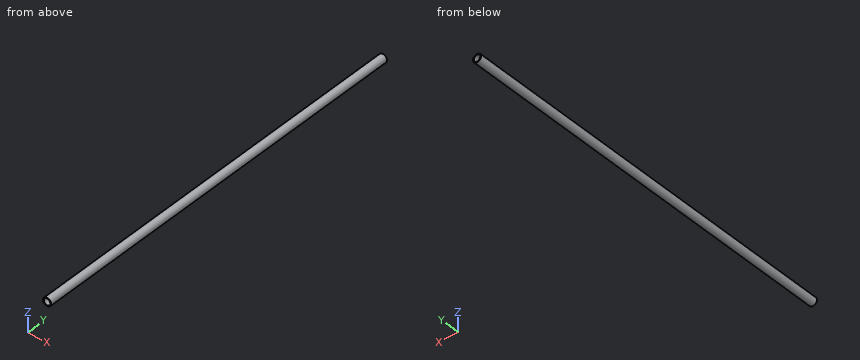
from build123d import *

# Parameters (mm, degrees)
CYLINDER_R          = 16.7005
CYLINDER_DEPTH      = 1609.72
CYLINDER_ROLL_ANGLE = 90
THICKNESS001_T      = -3.3782


with BuildPart() as part:
    # Cylinder → Cylinder (new body)
    with BuildSketch(Plane.XY):
        Circle(CYLINDER_R)
    extrude(amount=CYLINDER_DEPTH)


with BuildPart() as part_1:
    # Cylinder roll: moved
    add(part.part.rotate(Axis((0, 0, 0), (1, 0, 0)), CYLINDER_ROLL_ANGLE))


with BuildPart() as part_2:
    # Cylinder placement: moved
    add(part_1.part)

    # Thickness001
    thickness001_openings = [part_2.faces().sort_by_distance(p)[0] for p in [
        (0, 0, 0),
        (0, -1609.72, 0),
    ]]
    offset(amount=THICKNESS001_T, openings=thickness001_openings)


solid = part_2.part
Work out the finished part from the listing and answer in its coordinate system (mm). Round coordinates to 2 decimals unless told otherwise and drop trailing zeros. Order: outer loops, then holes, each group sorted by start corner. A loop starts at its lowest first (then second) coordinate and runs counter-clockwise, first axis right, second up. Notation, with made-up numbers: M -20.75,87.25 L 38.25,87.25 A14 ccw 38.25,92.25 Z; hole C -35,7.5 d2. An arc over 180 degrees is marked long. Put each result on its own line as item: value. Start each with the question number.
Q1. Straight lines are drawn through the part: L1, parallel to Z at x = 0, y = -679; L2, parallel to Z at x = -2.5, y = -1477; L3, parallel to X at y = -1381, z = 7. For each, find the intervals that lie inside material, in ascending order. Write a range as [from, to].
Q2. Flat-ended cylindrical pins translate along their axes: pin 1 (10 mm diameter, centred on x = 4, z = 2.5, fed in from +Y); pin 2 (12 mm diameter, centred on y = -988.5, z = -6.5, fed in from +X); pin 3 (2 mm diameter, centred on y = -500.5, z = -6, fed in from +X); pin 4 (5 mm diameter, centred on x = 12.5, y = -736, fed in from -Z). Find the tip coordinate at first contact, or state that the pin passes through.
Q3. Section C-C, the plane y = -813 is taken. Write down the section's boundary in (x, z).
Q4. Section B-B, the plane x = 0 is taken. Write down the section's boundary in (y, z).
Q5. Section A-A, the plane z = 0 is taken. Write down the section's boundary in (x, y).
Findings below:
1. L1: z = [-16.7, -13.32], [13.32, 16.7]
1. L2: z = [-16.51, -13.09], [13.09, 16.51]
1. L3: x = [-15.16, -11.34], [11.34, 15.16]
2. pin 1: passes through
2. pin 2: stops at x = 16.69
2. pin 3: stops at x = 15.93
2. pin 4: stops at z = -13.38
3. outline: C 0,0 d33.4; hole C 0,0 d26.64
4. outline: M -1609.72,-16.7 L 0,-16.7 L 0,-13.32 L -1609.72,-13.32 Z; M -1609.72,13.32 L 0,13.32 L 0,16.7 L -1609.72,16.7 Z
5. outline: M -16.7,-1609.72 L -13.32,-1609.72 L -13.32,0 L -16.7,0 Z; M 13.32,-1609.72 L 16.7,-1609.72 L 16.7,0 L 13.32,0 Z
